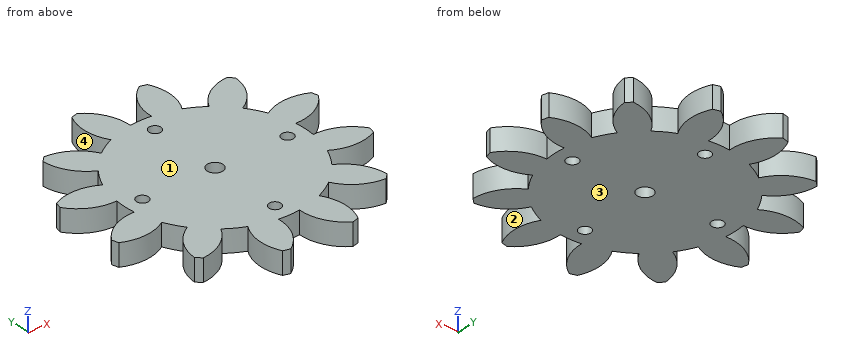
```python
from build123d import *

# Parameters (mm, degrees)
SKETCH1_R           = 0.83
BOSS_EXTRUDE1_DEPTH = 2.35
SKETCH2_R           = 0.625
CUT_EXTRUDE1_DEPTH  = 10
CIRPATTERN1_COUNT   = 4


with BuildPart() as part:
    # Sketch1 → Boss-Extrude1 (new body)
    with BuildSketch(Plane.XY):
        with BuildLine():
            ThreePointArc((31.089190509, -0.00961289), (28.777823425, -0.762116774), (27.131493603, -2.550489779))
            ThreePointArc((27.131493603, -2.550489779), (26.201203233, -1.937982234), (25.205610954, -1.438580913))
            ThreePointArc((25.205610954, -1.438580913), (25.931222497, 0.881369039), (25.427226435, 3.259323592))
            ThreePointArc((25.427226435, 3.259323592), (25.075169864, 3.358604023), (24.720639715, 3.448652933))
            ThreePointArc((24.720639715, 3.448652933), (23.095189045, 1.641281911), (22.563612099, -0.730659454))
            ThreePointArc((22.563612099, -0.730659454), (21.451703233, -0.665357545), (20.339794367, -0.730659454))
            ThreePointArc((20.339794367, -0.730659454), (19.80821742, 1.641281911), (18.182766751, 3.448652933))
            ThreePointArc((18.182766751, 3.448652933), (17.828236601, 3.358604023), (17.47618003, 3.259323592))
            ThreePointArc((17.47618003, 3.259323592), (16.972183969, 0.881369039), (17.697795512, -1.438580913))
            ThreePointArc((17.697795512, -1.438580913), (16.702203233, -1.937982234), (15.771912863, -2.550489779))
            ThreePointArc((15.771912863, -2.550489779), (14.12558304, -0.762116774), (11.814215957, -0.00961289))
            ThreePointArc((11.814215957, -0.00961289), (11.552208296, -0.264862608), (11.296958578, -0.526870269))
            ThreePointArc((11.296958578, -0.526870269), (12.049462462, -2.838237352), (13.837835467, -4.484567174))
            ThreePointArc((13.837835467, -4.484567174), (13.225327922, -5.414857545), (12.725926601, -6.410449824))
            ThreePointArc((12.725926601, -6.410449824), (10.40597665, -5.684838281), (8.028022096, -6.188834342))
            ThreePointArc((8.028022096, -6.188834342), (7.928741665, -6.540890913), (7.838692755, -6.895421063))
            ThreePointArc((7.838692755, -6.895421063), (9.646063777, -8.520871732), (12.018005142, -9.052448679))
            ThreePointArc((12.018005142, -9.052448679), (11.952703233, -10.164357545), (12.018005142, -11.276266411))
            ThreePointArc((12.018005142, -11.276266411), (9.646063777, -11.807843357), (7.838692755, -13.433294027))
            ThreePointArc((7.838692755, -13.433294027), (7.928741665, -13.787824176), (8.028022096, -14.139880747))
            ThreePointArc((8.028022096, -14.139880747), (10.40597665, -14.643876808), (12.725926601, -13.918265265))
            ThreePointArc((12.725926601, -13.918265265), (13.225327922, -14.913857545), (13.837835467, -15.844147915))
            ThreePointArc((13.837835467, -15.844147915), (12.049462462, -17.490477737), (11.296958578, -19.80184482))
            ThreePointArc((11.296958578, -19.80184482), (11.552208296, -20.063852481), (11.814215957, -20.3191022))
            ThreePointArc((11.814215957, -20.3191022), (14.12558304, -19.566598315), (15.771912863, -17.77822531))
            ThreePointArc((15.771912863, -17.77822531), (16.702203233, -18.390732855), (17.697795512, -18.890134176))
            ThreePointArc((17.697795512, -18.890134176), (16.972183969, -21.210084128), (17.47618003, -23.588038682))
            ThreePointArc((17.47618003, -23.588038682), (17.828236601, -23.687319113), (18.182766751, -23.777368023))
            ThreePointArc((18.182766751, -23.777368023), (19.80821742, -21.969997001), (20.339794367, -19.598055636))
            ThreePointArc((20.339794367, -19.598055636), (21.451703233, -19.663357545), (22.563612099, -19.598055636))
            ThreePointArc((22.563612099, -19.598055636), (23.095189045, -21.969997001), (24.720639715, -23.777368023))
            ThreePointArc((24.720639715, -23.777368023), (25.075169864, -23.687319113), (25.427226435, -23.588038682))
            ThreePointArc((25.427226435, -23.588038682), (25.931222497, -21.210084128), (25.205610954, -18.890134176))
            ThreePointArc((25.205610954, -18.890134176), (26.201203233, -18.390732855), (27.131493603, -17.77822531))
            ThreePointArc((27.131493603, -17.77822531), (28.777823425, -19.566598315), (31.089190509, -20.3191022))
            ThreePointArc((31.089190509, -20.3191022), (31.351198169, -20.063852481), (31.606447888, -19.80184482))
            ThreePointArc((31.606447888, -19.80184482), (30.853944004, -17.490477737), (29.065570998, -15.844147915))
            ThreePointArc((29.065570998, -15.844147915), (29.678078543, -14.913857545), (30.177479864, -13.918265265))
            ThreePointArc((30.177479864, -13.918265265), (32.497429816, -14.643876808), (34.87538437, -14.139880747))
            ThreePointArc((34.87538437, -14.139880747), (34.974664801, -13.787824176), (35.064713711, -13.433294027))
            ThreePointArc((35.064713711, -13.433294027), (33.257342689, -11.807843357), (30.885401324, -11.276266411))
            ThreePointArc((30.885401324, -11.276266411), (30.950703233, -10.164357545), (30.885401324, -9.052448679))
            ThreePointArc((30.885401324, -9.052448679), (33.257342689, -8.520871732), (35.064713711, -6.895421063))
            ThreePointArc((35.064713711, -6.895421063), (34.974664801, -6.540890913), (34.87538437, -6.188834342))
            ThreePointArc((34.87538437, -6.188834342), (32.497429816, -5.684838281), (30.177479864, -6.410449824))
            ThreePointArc((30.177479864, -6.410449824), (29.678078543, -5.414857545), (29.065570998, -4.484567174))
            ThreePointArc((29.065570998, -4.484567174), (30.853944004, -2.838237352), (31.606447888, -0.526870269))
            ThreePointArc((31.606447888, -0.526870269), (31.351198169, -0.264862608), (31.089190509, -0.00961289))
        make_face()
        with Locations((21.451703233, -10.164357545)):
            Circle(SKETCH1_R, mode=Mode.SUBTRACT)
    extrude(amount=BOSS_EXTRUDE1_DEPTH)

    # Sketch2 → Cut-Extrude1 (cut)
    with BuildSketch(Plane.XY.offset(2.35)):
        with Locations((21.451703233, -2.514357545)):
            Circle(SKETCH2_R)
    cut_extrude1 = extrude(amount=-CUT_EXTRUDE1_DEPTH, mode=Mode.SUBTRACT)

    # CirPattern1: Cut-Extrude1 ×4 about axis
    cirpattern1_axis = Axis((21.451703233, -10.164357545, 0), (0, 0, 1))
    for i in range(1, CIRPATTERN1_COUNT):
        add(cut_extrude1.rotate(cirpattern1_axis, i * 360 / CIRPATTERN1_COUNT), mode=Mode.SUBTRACT)


solid = part.part
```
Geometry: final body of the model. Coordinates: model frame, mm. Face numbers are marked on the shaded views. A direction names the side the tool comes from. Round coordinates to 2 decimals unless told otherwise and drop trailing zeros. Order: outer loops, then holes, each group sorted by start corner. A loop starts at its lowest first (then second) coordinate and runs counter-clockwise, first axis right, second up. Notation, with made-up numbers: (24.25, 28.25) -> (59.25, 28.25) arc R24 ccw to (59.25, 52.25) -> close; hole circle Ø10 at (37, -19.75). An arc over 180 degrees is marked (long way). Use one line per item in the form item = value.
(1) Ray query, probe 1 along X at (y, z) = (-10.25, 0.7); probe 2 along X at (y, z) = (-1, 0.3); probe 3 along Y at (x, z) = (21.75, 1.5). Return the intervals inside material, ascending. Write a range as [from, to].
Results list:
probe_1 = [11.95, 13.18], [14.42, 20.63], [22.28, 28.48], [29.72, 30.95]
probe_2 = [11.35, 14.46], [17.45, 25.45], [28.44, 31.55]
probe_3 = [-19.66, -18.36], [-17.27, -10.94], [-9.39, -3.06], [-1.97, -0.67]
(2) Section A-A on z = 0.95. Count the separate pieces of the cut face and the enclosed holes in it, and give its area (3 significant figures).
Results list:
separate_pieces = 1
enclosed_holes = 5
area = 417 mm^2
(3) Access query for the marked faces 3 and 4. Directions: +Z, -Z, +X, -X, +Y, -Y. A direction counts if a zero-diameter tool reaches every point of the face in a straight line with its end or side. Return the directions, or none.
Results list:
face_3 = -Z, +X, -X, +Y, -Y
face_4 = +Z, -Z
(4) Section C-C on x = 19. Return loops of the section in (y, z), and give its area (3 significant figures).
Results list:
outline = (-23.1, 0) -> (2.77, 0) -> (2.77, 2.35) -> (-23.1, 2.35) -> close
area = 60.8 mm^2
(5) Draft query along Y for the marked faces 1 and 2. Return one class per face: pulls with the +Y half, pulls with the -Y half, needs draft (parallel to the pull), parting line crosses it, or undercut.
Results list:
face_1 = needs draft
face_2 = undercut
(6) First-contact query: pin 1 Ø1.1 at (x, y) = (21.45, -2.51) entering from +Z. Flat tip, straight axial feed; report the tip coordinate or a pass-through.
Results list:
pin_1 = through
(7) Section B-B on x = 27.75. Return loops of the section in (y, z).
Results list:
outline = (-18.68, 0) -> (-1.65, 0) -> (-1.65, 2.35) -> (-18.68, 2.35) -> close
